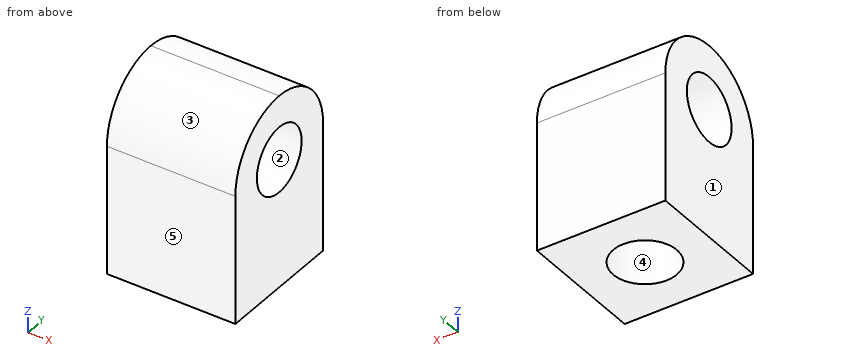
```python
from build123d import *

# Parameters (mm, degrees)
SKETCH1_W           = 10
SKETCH1_H           = 10
SKETCH1_R           = 2.475
BOSS_EXTRUDE2_DEPTH = 15
SKETCH2_R           = 2.55
CUT_EXTRUDE1_DEPTH  = 10
FILLET1_R           = 5
SKETCH1_5_R         = 2.475
CUT_EXTRUDE2_DEPTH  = 7


with BuildPart() as part:
    # Sketch1 → Boss-Extrude2 (new body)
    # profile 1 of 2: a face of its own
    with BuildSketch(Plane.XY):
        Rectangle(SKETCH1_W, SKETCH1_H)
        Circle(SKETCH1_R, mode=Mode.SUBTRACT)
    # profile 2 of 2: a face of its own
    with BuildSketch(Plane.XY):
        Circle(SKETCH1_R)
    extrude(amount=BOSS_EXTRUDE2_DEPTH)

    # Sketch2 → Cut-Extrude1 (cut)
    with BuildSketch(Plane.ZY.offset(5)):
        with Locations((10, 0)):
            Circle(SKETCH2_R)
    extrude(amount=-CUT_EXTRUDE1_DEPTH, mode=Mode.SUBTRACT)

    # Fillet1
    fillet1_edges = [part.edges().sort_by_distance(p)[0] for p in [
        (0, -5, 15),
        (0, 5, 15),
    ]]
    fillet(fillet1_edges, radius=FILLET1_R - 0.0001)  # a hair under: the kernel refuses the full size

    # Sketch1<5> → Cut-Extrude2 (cut)
    with BuildSketch(Plane.XY):
        Circle(SKETCH1_5_R)
    extrude(amount=CUT_EXTRUDE2_DEPTH, mode=Mode.SUBTRACT)


solid = part.part
```
CAD build for the part. Positions are in the model's coordinates, mm. Face numbers are marked on the shaded views. A direction names the side the tool comes from. Give positions to 0.01 mm unless a question says otherwise; leave off trailing zeros. Loops run counter-clockwise (first coordinate to the right, second up) from the corner with the lowest first, then second, coordinate; pieces in that order, holes last. Notation, with made-up numbers: M -20.75,17.5 L 6.25,17.5 A33 cw 6.25,48.5 Z; hole C 50.5,39.5 d10. An arc over 180 degrees is marked long. Use one line per item in the form item = value.
Item 1: Slice it at A-A (y = 1.5). List the corners of the cut face in (x, z).
Determined:
outline = M -5,0 L -1.97,0 L -1.97,7 L 1.97,7 L 1.97,0 L 5,0 L 5,7.94 L -5,7.94 Z; M -5,12.06 L 5,12.06 L 5,14.77 L -5,14.77 Z
Item 2: Flat gauge pins, fed straight in: pin 1 (1.5 mm diameter, centred on x = -3, y = 2.5, fed in from +Z); pin 2 (1 mm diameter, centred on x = -2, y = -1.5, fed in from +Z); pin 3 (1.5 mm diameter, centred on x = 0.5, y = -1, fed in from -Z). Where does each tip first touch, or does it go through?
Determined:
pin_1 = 14.68
pin_2 = 14.9
pin_3 = 7
Item 3: Which spindle directions (+Z, -Z, +X, -X, +Y, -Y) get a long thin tool onto all of the face, cutting with end or side? Do the marked faces 4 and 5. Say none if no direction does.
Determined:
face_4 = -Z
face_5 = +Z, -Z, +X, -X, -Y
Item 4: Two-plate mould, pull along Z, no slides. Class the marked faces 1, 2 and 3: pulls with the +Z half, pulls with the -Z half, needs draft (parallel to the pull), parting line crosses it, or undercut.
Determined:
face_1 = needs draft
face_2 = undercut
face_3 = pulls with the +Z half
Item 5: Slice it at D-D (z = 11). List the corners of the cut face in (x, y), plus the area to 3 significant figures.
Determined:
outline = M -5,-4.9 L 5,-4.9 L 5,-2.35 L -5,-2.35 Z; M -5,2.35 L 5,2.35 L 5,4.9 L -5,4.9 Z
area = 51.1 mm2
Item 6: Slice it at C-C (z = 3). List the corners of the cut face in (x, y) (3 decimals).
Determined:
outline = M -5,-5 L 5,-5 L 5,5 L -5,5 Z; hole C 0,0 d4.95
Item 7: Drill centre lines: probe 1 along Y at (x, z) = (0, 4) (3 decimals); probe 2 along Y at (x, z) = (-4.5, 11); probe 3 along X at (y, z) = (-0.75, 4). Where is each one in solid material? Low to high. Write a range as from..to.
Determined:
probe_1 = -5..-2.475, 2.475..5
probe_2 = -4.9..-2.35, 2.35..4.9
probe_3 = -5..-2.36, 2.36..5
